```python
from build123d import *

# Parameters (mm, degrees)
F0_W      = 50.8
F0_H      = 101.6
F1_DEPTH  = 12.7
F2_W      = 19.05
F2_H      = 50.8
F3_DEPTH  = 44.45
F5_DEPTH  = 25.4
F6_W      = 31.75
F6_H      = 9.652
F7_DEPTH  = 44.45
F8_SIZE2  = 31.7503775051
F8_SIZE   = 44.45
F9_R      = 11.176
F10_DEPTH = 25.4


with BuildPart() as f1:
    # F0 (on Top) → F1 (new body)
    with BuildSketch(Plane.XY):
        with Locations((5.7387277484, 35.3047995863)):
            Rectangle(F0_W, F0_H)
    extrude(amount=F1_DEPTH)

    # F2 (on face) → F3 (join)
    with BuildSketch(Plane.XY.offset(12.7)):
        with Locations((-10.1362722516, 60.7047995863)):
            Rectangle(F2_W, F2_H)
    extrude(amount=F3_DEPTH)

    # F4 (on face) → F5 (cut)
    with BuildSketch(Plane.XY.offset(12.7)):
        with BuildLine():
            Line((-2.1200233605, 16.0007995863), (-2.1200233605, 0.2527995863))
            ThreePointArc((-2.1200233605, 0.2527995863), (5.7539766395, -7.6212004137), (13.6279766395, 0.2527995863))
            Line((13.6279766395, 0.2527995863), (13.6279766395, 16.0007995863))
            ThreePointArc((13.6279766395, 16.0007995863), (5.7539766395, 23.8747995863), (-2.1200233605, 16.0007995863))
        make_face()
    extrude(amount=-F5_DEPTH, mode=Mode.SUBTRACT)

    # F6 (on face) → F7 (join)
    with BuildSketch(Plane.XY.offset(12.7)):
        with Locations((15.2637277484, 81.2787995863)):
            Rectangle(F6_W, F6_H)
    extrude(amount=F7_DEPTH)

    # F8
    f8_edges = [f1.edges().sort_by_distance(p)[0] for p in [
        (31.138728, 81.2788, 57.15),
    ]]
    f8_side = f1.faces().sort_by_distance((31.138728, -14.329495, 6.35))[0]
    chamfer(f8_edges, length=F8_SIZE, length2=F8_SIZE2, reference=f8_side)

    # F9 (on face) → F10 (cut)
    with BuildSketch(Plane.YZ.offset(-0.6112722516)):
        with Locations((55.8787995863, 34.798)):
            Circle(F9_R)
    extrude(amount=-F10_DEPTH, mode=Mode.SUBTRACT)


solid = f1.part
```
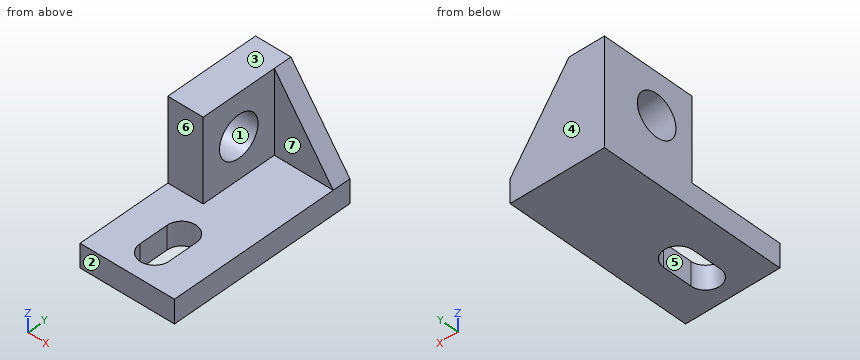
Check sheet for the modelled part. Datum: model origin and axes. Units: mm. Face numbers are marked on the shaded views. A direction names the side the tool comes from. Give positions to 0.01 mm unless a question says otherwise; leave off trailing zeros. Write each loop counter-clockwise with the first axis right and the second up, starting at its lowest first coordinate (ties: lowest second). Pieces come first, ordered by that corner, then holes. Notation, with made-up numbers: (-8.75, 87) -> (48.25, 87) arc R11 cw to (48.25, 106) -> close; hole circle Ø9 at (14.5, 49.25). An arc over 180 degrees is marked (long way). Use CSV: the item, a comma, the result in double quotes. Start each with the question number.
Q1. Cross-section at C-C on x = 6.5. Enter the section's corners in (y, z).
Q2. Tool access check on the marked faces 4, 5, 6 and 7. Record the directions out of +Z, -Z, +X, -X, +Y, -Y that give a thin tool (end or side, any length) a straight path to the whole face; none if there is none.
Q3. Release check for a two-part mould opening along Z. For the marked faces 1, 2 and 3 record: +Z half, -Z half, draft (parallel to the pull), parting line (faces both ways), or undercut.
Q4. Depth check by flat-ended pin: P1, Ø18, axis at y = 55.88, z = 34.8, coming from the +X side; P2, Ø9.5, axis at x = 11, z = 34, coming from the -Y side; P3, Ø5.5, axis at x = -12.5, z = 35, coming from the -Y side; P4, Ø12.5, axis at y = 60.5, z = 41.5, coming from the +X side. Enter the tip coordinate at first touch or a pass-through.
Q5. Cross-section at B-B on z = 8. Enter the section's corners in (x, y), and give its area (3 significant figures).
Q6. Scan lines: line 1 along X through (y, z) = (36, 52); line 2 along Z through (x, y) = (12, 21.5); line 3 along Y through (x, z) = (19, 27). Record each from-to range of solid material in increasing order.
Q7. Cross-section at D-D on z = 40. Enter the section's corners in (x, y), and give its area (3 significant figures).
Q8. Cross-section at A-A on y = 14. Enter the section's corners in (x, z).
Working result:
1,outline,"(-15.5, 0) -> (-7.59, 0) -> (-7.59, 12.7) -> (-15.5, 12.7) -> close; (23.84, 0) -> (86.1, 0) -> (86.1, 47.19) -> (76.45, 47.19) -> (76.45, 12.7) -> (23.84, 12.7) -> close"
2,face 4,"+Z, -Z, +X, -X, +Y"
2,face 5,"+Z, -Z"
2,face 6,"+Z, +X, -X, -Y"
2,face 7,"+Z, +X, -Y"
3,face 1,"undercut"
3,face 2,"draft"
3,face 3,"+Z half"
4,P1,"passes through"
4,P2,"stops at y = 76.45"
4,P3,"stops at y = 35.3"
4,P4,"stops at x = -0.61"
5,outline,"(-19.66, -15.5) -> (31.14, -15.5) -> (31.14, 86.1) -> (-19.66, 86.1) -> close; hole (-2.12, 0.25) arc R7.87 ccw to (13.63, 0.25) -> (13.63, 16) arc R7.87 ccw to (-2.12, 16) -> close"
5,area,"4,720 mm^2"
6,line 1,"x = -19.66 to -0.61"
6,line 2,"z = 0 to 12.7"
6,line 3,"y = 76.45 to 86.1"
7,outline,"(-19.66, 35.3) -> (-0.61, 35.3) -> (-0.61, 45.99) -> (-19.66, 45.99) -> close; (-19.66, 65.77) -> (-0.61, 65.77) -> (-0.61, 76.45) -> (11.64, 76.45) -> (11.64, 86.1) -> (-19.66, 86.1) -> close"
7,area,"709 mm^2"
8,outline,"(-19.66, 0) -> (-2.12, 0) -> (-2.12, 12.7) -> (-19.66, 12.7) -> close; (13.63, 0) -> (31.14, 0) -> (31.14, 12.7) -> (13.63, 12.7) -> close"
